Model file for the job. Use its own axes, mm. A direction names the side the tool comes from. Give positions to 0.01 mm unless a question says otherwise; leave off trailing zeros. Loops run counter-clockwise (first coordinate to the right, second up) from the corner with the lowest first, then second, coordinate; pieces in that order, holes last. Notation, with made-up numbers: M 58.5,56 L 80.5,56 A28 ccw 80.5,93 Z; hole C 67.25,49 d6. An arc over 180 degrees is marked long. Use CSV: the item, a comma, the result in double quotes. Start each with the question number.
(1) Wall check: line 1 along X through (y, z) = (-5.25, 0.6); line 2 along X through (y, z) = (-7.25, 0.1); line 3 along Y through (x, z) = (-0.6, -0.5). Give the ranges that are in metal, low to high. Write a range as from..to.
(2) Two-plate mould, pull along X, no slides. Class faces 1 (the face through (2.78, 0.25, 0.62)), 2 (the face through (0, 0, -2)), 3 (the face through (1, 1, 0)): pulls with the +X half, pulls with the -X half, needs draft (parallel to the pull), parting line crosses it, or undercut.
(3) Slice it at A-A on y = -7.5. List the corners of the cut face in (x, z).
(4) Flat gauge pins, fed straight in: P1, Ø0.9, axis at y = 1, z = 0, coming from the +X side; P2, Ø1.5, axis at y = -5, z = -1, coming from the -X side; P3, Ø0.6, axis at y = 1, z = 0, coming from the -X side. Where does each tip first touch, or does it go through?
(5) Tool access for faces 4 (the face through (0, -12, 0)), 5 (the face through (-0.45, -6.01, -1.43)), 6 (the face through (-0.51, 1.11, 0.86)): list every direction of +Z, -Z, +X, -X, +Y, -Y with a clear straight run to the whole face (end or side of a thin tool).
```python
from build123d import *

# Parameters (mm, degrees)
CUT_EXTRUDE1_DEPTH = 1.1


with BuildPart() as part:
    # Sketch1 → Revolve1 (revolve)
    with BuildSketch(Plane.XY, mode=Mode.PRIVATE) as revolve1_sk:
        with BuildLine():
            Line((-1.5, -0.1), (-1.5, -11.75))
            Line((-1.5, -11.75), (-1.25, -12))
            Line((-1.25, -12), (0, -12))
            Line((0, -12), (0, 1.65))
            Line((0, 1.65), (-1.372450351, 1.65))
            ThreePointArc((-1.372450351, 1.65), (-1.400779398, 1.648389744), (-1.42874351, 1.643579721))
            ThreePointArc((-1.42874351, 1.643579721), (-2.295395633, 1.200105689), (-2.85, 0.4))
            Line((-2.85, 0.4), (-2.85, 0.1))
            ThreePointArc((-2.85, 0.1), (-2.820710678, 0.029289322), (-2.75, 0))
            Line((-2.75, 0), (-1.6, 0))
            ThreePointArc((-1.6, 0), (-1.529289322, -0.029289322), (-1.5, -0.1))
        make_face()
    revolve(revolve1_sk.sketch.rotate(Axis((0, -12, 0), (0, 1, 0)), 270), axis=Axis((0, -12, 0), (0, 1, 0)))

    # Sketch2 → Cut-Extrude1 (cut)
    with BuildSketch(Plane(origin=(0, 1.65, 0), x_dir=(1, 0, 0), z_dir=(0, 1, 0))):
        Polygon((-1, 0.577350269), (-1, -0.577350269), (0, -1.154700538), (1, -0.577350269), (1, 0.577350269), (0, 1.154700538), align=None)
    extrude(amount=-CUT_EXTRUDE1_DEPTH, mode=Mode.SUBTRACT)


solid = part.part
```
Reply:
1,line 1,"x = -1.37..1.37"
1,line 2,"x = -1.5..1.5"
1,line 3,"y = -12..0.55"
2,face 1,"parting line crosses it"
2,face 2,"needs draft"
2,face 3,"undercut"
3,outline,"C 0,0 d3"
4,P1,"stops at x = 2.79"
4,P2,"stops at x = -1.48"
4,P3,"stops at x = -2.71"
5,face 4,"+Z, -Z, +X, -X, -Y"
5,face 5,"-Y"
5,face 6,"+Y"
